Input: part model. Units: mm. Frame: model coordinates. Face numbers are marked on the shaded views. A direction names the side the tool comes from. Round coordinates to 2 decimals unless told otherwise and drop trailing zeros. Order: outer loops, then holes, each group sorted by start corner. A loop starts at its lowest first (then second) coordinate and runs counter-clockwise, first axis right, second up. Notation, with made-up numbers: (67.25, 68) -> (101.25, 68) arc R18 ccw to (101.25, 101) -> close; hole circle Ø5 at (34.25, 23.5). An arc over 180 degrees is marked (long way). Answer as CSV lines item,"result". Start each with the question number.
1) Mould query, pull axis Y, two halves, no side actions, for the marked faces 5, 6 and 7. Classes: +Y half, -Y half, draft (parallel to the pull), parting line (faces both ways), or undercut.
2) Section query C-C, the plane x = 83. Output: boundary loops of the cut face in (y, z), and give its area (3 significant figures).
3) Section query B-B, the plane y = 179.5. Output: boundary loops of the cut face in (x, z), and give its area (3 significant figures).
4) Line query: L1, parallel to X at y = -257.5, z = 433.5; L2, parallel to X at y = 143, z = 116.5; L3, parallel to Z at x = -319.5, y = -261. Output: solid intervals per line, ascending.
5) Access query for the marked faces 1, 2, 3 and 4. Directions: +Z, -Z, +X, -X, +Y, -Y. A direction counts if a zero-diameter tool reaches every point of the face in a straight line with its end or side. Return the directions, or none.
6) First-contact query: P1, Ø3, axis at x = -363.5, y = 189, coming from the +Z side; P2, Ø5, axis at x = -124, z = 2.5, coming from the -Y side; P3, Ø5, axis at x = 44.5, y = 137, coming from the -Z side. Flat tips, straight axial feed; report the tip coordinate or a pass-through.
7) Section query A-A, the plane z = 262. Output: boundary loops of the cut face in (x, y).
```python
from build123d import *

# Parameters (mm, degrees)
F0_W     = 1000
F0_H     = 500
F1_DEPTH = 464
F2_W     = 980
F2_H     = 480
F3_DEPTH = 10
F4_T     = -10
F5_W     = 1000
F5_H     = 50
F6_DEPTH = 15
F8_D     = 6
F8_DEPTH = 15
F8_TIP   = 1.8025818571


# Not quite as in the source:
# - a shell that OpenCascade refuses in one call is made with other operations: the cavity is built on its own and cut out


with BuildPart() as f1:
    # F0 (on Top) → F1 (new body)
    with BuildSketch(Plane.XY):
        Rectangle(F0_W, F0_H)
    extrude(amount=F1_DEPTH)

    # F2 (on face) → F3 (cut)
    with BuildSketch(Plane(origin=(0, 0, 0), x_dir=(1, 0, 0), z_dir=(0, 0, -1))):
        Rectangle(F2_W, F2_H)
    extrude(amount=-F3_DEPTH, mode=Mode.SUBTRACT)

    # F4: a shell. OpenCascade refuses it in one call, so the cavity is built on its own and cut out:
    # the body offset inwards by the wall thickness, plus a prism from it out through each open face.
    f4_core = offset(f1.part, amount=F4_T, kind=Kind.INTERSECTION, mode=Mode.PRIVATE)
    f4_exits = [f4_core.faces().sort_by_distance(p)[0] for p in [
        (0, 0, 454),
    ]]
    add(f4_core, mode=Mode.SUBTRACT)
    extrude(f4_exits, amount=-F4_T, mode=Mode.SUBTRACT)

    # F5 (on face) → F6 (join)
    with BuildSketch(Plane.XZ.offset(250)):
        with Locations((0, 424)):
            Rectangle(F5_W, F5_H)
    extrude(amount=F6_DEPTH)

    # F8
    with Locations(Plane.XZ.offset(265)):
        with Locations((-350, 433.5), (-319.5, 433.5), (319.5, 433.5), (350, 433.5)):
            Hole(F8_D / 2, depth=F8_DEPTH)
            with Locations((0, 0, -(F8_DEPTH + F8_TIP / 2))):  # 118° drill point
                Cone(0, F8_D / 2, F8_TIP, mode=Mode.SUBTRACT)


solid = f1.part
```
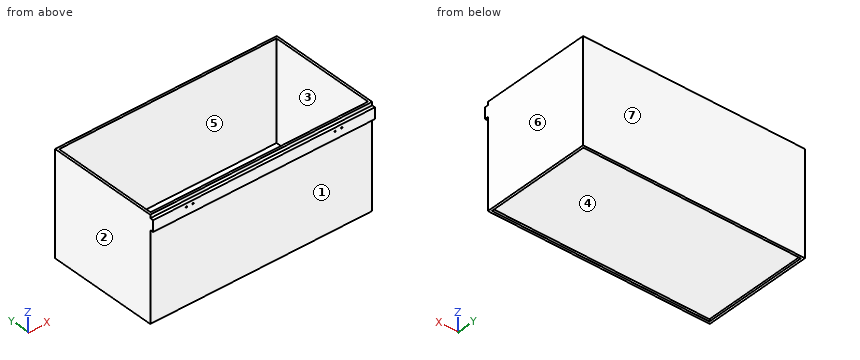
Findings:
1,face 5,"undercut"
1,face 6,"draft"
1,face 7,"+Y half"
2,outline,"(-265, 399) -> (-250, 399) -> (-250, 0) -> (-240, 0) -> (-240, 10) -> (240, 10) -> (240, 0) -> (250, 0) -> (250, 464) -> (240, 464) -> (240, 20) -> (-240, 20) -> (-240, 464) -> (-250, 464) -> (-250, 449) -> (-265, 449) -> close"
2,area,"14,800 mm^2"
3,outline,"(-500, 0) -> (-490, 0) -> (-490, 10) -> (490, 10) -> (490, 0) -> (500, 0) -> (500, 464) -> (490, 464) -> (490, 20) -> (-490, 20) -> (-490, 464) -> (-500, 464) -> close"
3,area,"19,100 mm^2"
4,L1,"x = -500 to -353, -347 to -322.5, -316.5 to 316.5, 322.5 to 347, 353 to 500"
4,L2,"x = -500 to -490, 490 to 500"
4,L3,"z = 399 to 430.5, 436.5 to 449"
5,face 1,"-Z, +X, -X, -Y"
5,face 2,"+Z, -Z, -X, +Y, -Y"
5,face 3,"+Z"
5,face 4,"-Z"
6,P1,"stops at z = 20"
6,P2,"stops at y = -250"
6,P3,"stops at z = 10"
7,outline,"(-500, -250) -> (500, -250) -> (500, 250) -> (-500, 250) -> close; hole (-490, -240) -> (490, -240) -> (490, 240) -> (-490, 240) -> close"
